Input: part model. Units: mm. Frame: model coordinates. Round coordinates to 2 decimals unless told otherwise and drop trailing zeros. Loops run counter-clockwise (first coordinate to the right, second up) from the corner with the lowest first, then second, coordinate; pieces in that order, holes last. Notation, with made-up numbers: (60, 41.5) -> (103, 41.5) arc R15 cw to (103, 67.5) -> close; hole circle Ø9 at (-6.75, 63.25). An arc over 180 degrees is marked (long way). Answer as a JSON object with one key per item and string values. Group by question number.
Item 1: Section query A-A on z = 47. Return loops of the section in (x, y).
Item 2: Pin query (flat end, axial travel): pin 1 (6 mm diameter, centred on x = 14, z = 103.5, fed in from -Y). Return the tip coordinate at first contact, or that it passes through.
Item 3: Draft query along X for faces 1 (the cylindrical face through (21.566, 0.108, 30.42)), 2 (the flat face through (14, -3, 0)), 3 (the cylindrical face through (21.25, -5.16, 30.42)). Return one class per face: released by +X, released by -X, zero draft, split by the parting line, or undercut.
Item 4: Material intervals for line 1 (Y direction, x = 30, z = 117.5); line 2 (Y direction, x = 16.5, z = 67); line 3 (X direction, y = -5, z = 39), sorted ascending. Write a range as [from, to].
from build123d import *


with BuildPart() as f4:
    # F0 (on Top) → F4 section 0
    with BuildSketch(Plane.XY):
        with BuildLine():
            ThreePointArc((1.5474857793, -7.3085332362), (21.5310263119, -5.1508726081), (41.6096189935, -6.0714743331))
            ThreePointArc((41.6096189935, -6.0714743331), (21.2699883307, 0.1522717061), (0, 0))
            ThreePointArc((0, 0), (-3.2423450763, -4.5046204189), (1.5474857793, -7.3085332362))
        make_face()
    # F2 (on offset) → F4 section 1
    with BuildSketch(Plane.XY.offset(60)):
        with BuildLine():
            ThreePointArc((41.6096189935, -6.0714743331), (21.2699883307, 0.1522717061), (0, 0))
            ThreePointArc((0, 0), (-3.2423450763, -4.5046204189), (1.5474857793, -7.3085332362))
            ThreePointArc((1.5474857793, -7.3085332362), (21.5310263119, -5.1508726081), (41.6096189935, -6.0714743331))
        make_face()
    loft()

    # F4_face (on face) → F6 section 0
    with BuildSketch(Plane(origin=(14.0442099137, -3.0045587038, 60), x_dir=(1, 0, 0), z_dir=(0, 0, 1))):
        with BuildLine():
            ThreePointArc((-14.0442099137, 3.0045587038), (-17.28655499, -1.5000617151), (-12.4967241344, -4.3039745324))
            ThreePointArc((-12.4967241344, -4.3039745324), (7.4868163983, -2.1463139043), (27.5654090798, -3.0669156292))
            ThreePointArc((27.5654090798, -3.0669156292), (7.225778417, 3.1568304099), (-14.0442099137, 3.0045587038))
        make_face()
    # F5 (on offset) → F6 section 1
    with BuildSketch(Plane.XY.offset(130)):
        with BuildLine():
            ThreePointArc((23.7320419401, -4.9977814779), (32.6341024887, -5.3520079811), (41.5212251246, -5.97747555))
            ThreePointArc((41.5212251246, -5.97747555), (33.2689677889, -2.4114002007), (24.6086101979, 0))
            ThreePointArc((24.6086101979, 0), (22.2217339207, -2.1571242907), (23.7320419401, -4.9977814779))
        make_face()
    loft()


solid = f4.part
Solved:
{
 "1": {"outline": "(0, 0) arc R3.75 ccw (long way) to (1.55, -7.31) arc R131.18 cw to (41.61, -6.07) arc R70.22 ccw to start"},
 "2": {"pin 1": "y = -5.97"},
 "3": {"face 1": "split by the parting line", "face 2": "zero draft", "face 3": "undercut"},
 "4": {"line 1": "[-5.3, -1.65]", "line 2": "[-5.48, 0.55]", "line 3": "[-3.1, 39.28]"}
}
